Could you check a few things on this model? Use its own coordinates, in mm. Face numbers are marked on the shaded views. A direction names the side the tool comes from. Give positions to 0.01 mm unless a question says otherwise; leave off trailing zeros. Write each loop counter-clockwise with the first axis right and the second up, starting at its lowest first coordinate (ties: lowest second). Pieces come first, ordered by that corner, then holes. Notation, with made-up numbers: (26, 13) -> (30, 13) arc R23 ccw to (30, 44) -> close; hole circle Ø2 at (33, 63). An arc over 180 degrees is marked (long way). Write item = value, one per line. Start each with the question number.
```python
from build123d import *

# Parameters (mm, degrees)
F1_DEPTH = 26.67
F2_W     = 16
F2_H     = 2
F3_DEPTH = 20.32
F4_R     = 1.175
F5_DEPTH = 3


with BuildPart() as f1:
    # F0 (on Front) → F1 (new body)
    with BuildSketch(Plane.XZ):
        with BuildLine():
            ThreePointArc((-10.16, -3.7), (0, -1.7), (10.16, -3.7))
            Line((10.16, -3.7), (10.16, 2.3))
            Line((10.16, 2.3), (-10.16, 2.3))
            Line((-10.16, 2.3), (-10.16, -3.7))
        make_face()
    extrude(amount=F1_DEPTH)

    # F2 (on face) → F3 (cut, through all)
    with BuildSketch(Plane.YZ.offset(10.16)):
        with Locations((-13.335, 0)):
            Rectangle(F2_W, F2_H)
    extrude(amount=-F3_DEPTH, mode=Mode.SUBTRACT)

    # F4 (on face) → F5 (join)
    with BuildSketch(Plane.XY.offset(2.3)):
        with Locations((7.62, -2.54)):
            Circle(F4_R)
        with Locations((7.62, -24.13)):
            Circle(F4_R)
        with Locations((-7.62, -2.54)):
            Circle(F4_R)
        with Locations((-7.62, -24.13)):
            Circle(F4_R)
    extrude(amount=F5_DEPTH)


solid = f1.part
```
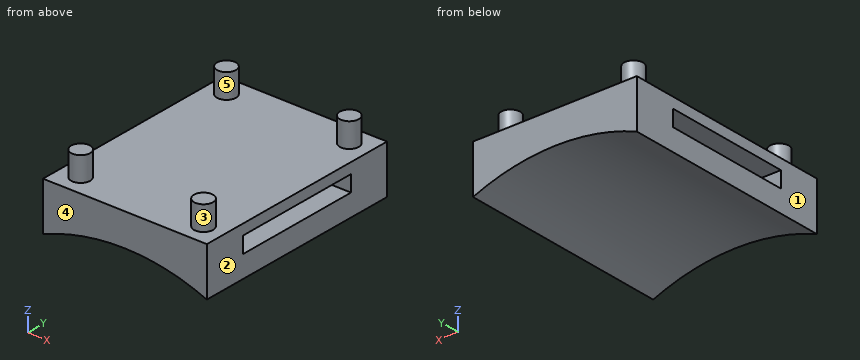
(1) I'm going to push flat-ended pins straight in: pin 1 (6 mm diameter, centred on x = 6.5, y = -13.5, fed in from +Z); pin 2 (6 mm diameter, centred on x = 7.5, y = -9.5, fed in from -Z). Where does each tip first touch, or does it pass through?
(2) If I drill on line 1 along Y through (x, z) = (8.75, 0) (3 decimals); line 2 along Z through (x, y) = (-4, -7.75); line 3 along Z through (x, y) = (4.5, -6), over which ranges is the centre line in solid material (lowest first)? Write a range as from..to.
(3) Imagine slicing it at C-C (y = -2.54). Please give me the cut outline in (x, z) (3 decimals), then the cut area to 3 significant figures.
(4) Imagine slicing it at A-A (z = 0). Please give me the cut outline in (x, y) (3 decimals), then the cut area to 3 significant figures.
(5) We'd pull the mould along X, two halves only. Please class the marked faces 1, 2 and 3: released by +X, released by -X, zero draft, split by the parting line, or undercut.
(6) Imagine slicing it at D-D (x = 1.25). Please give me the cut outline in (y, z) (3 decimals), then the cut area to 3 significant figures.
(7) On a 3-axis mill with a long thin cutter (end or side, diameter ignored), from which of +Z, -Z, +X, -X, +Y, -Y can I reach the whole of each face in a straight line? I mean the marked faces 4 and 5. Say none if no direction works.
(8) Imagine slicing it at B-B (y = -20.75). Please give me the cut outline in (x, z), then the cut area to 3 significant figures.
Answers below:
q1.pin_1 = 2.3
q1.pin_2 = -3.7
q2.line_1 = -26.67..-21.335, -5.335..0
q2.line_2 = -2..-1, 1..2.3
q2.line_3 = -2.08..-1, 1..2.3
q3.outline = (-10.16, -3.7) arc R26.806 cw to (10.16, -3.7) -> (10.16, 2.3) -> (8.795, 2.3) -> (8.795, 5.3) -> (6.445, 5.3) -> (6.445, 2.3) -> (-6.445, 2.3) -> (-6.445, 5.3) -> (-8.795, 5.3) -> (-8.795, 2.3) -> (-10.16, 2.3) -> close
q3.area = 109 mm^2
q4.outline = (-10.16, -26.67) -> (10.16, -26.67) -> (10.16, -21.335) -> (-10.16, -21.335) -> close; (-10.16, -5.335) -> (10.16, -5.335) -> (10.16, 0) -> (-10.16, 0) -> close
q4.area = 217 mm^2
q5.face_1 = released by -X
q5.face_2 = released by +X
q5.face_3 = undercut
q6.outline = (-26.67, -1.729) -> (0, -1.729) -> (0, 2.3) -> (-26.67, 2.3) -> close; hole (-21.335, -1) -> (-5.335, -1) -> (-5.335, 1) -> (-21.335, 1) -> close
q6.area = 75.5 mm^2
q7.face_4 = +Z, -Z, +X, -X, -Y
q7.face_5 = +Z
q8.outline = (-10.16, -3.7) arc R26.81 cw to (10.16, -3.7) -> (10.16, -1) -> (-10.16, -1) -> close; (-10.16, 1) -> (10.16, 1) -> (10.16, 2.3) -> (-10.16, 2.3) -> close
q8.area = 54.0 mm^2
